Verification items for the finished model (mm, model axes). A direction names the side the tool comes from. Round coordinates to 2 decimals unless told otherwise and drop trailing zeros. Order: outer loops, then holes, each group sorted by start corner. A loop starts at its lowest first (then second) coordinate and runs counter-clockwise, first axis right, second up. Notation, with made-up numbers: (-11, 62.5) -> (-2, 62.5) arc R27 cw to (-2, 83.5) -> close; hole circle Ø5 at (40, 27.5). An arc over 180 degrees is marked (long way). Answer in a Markdown table with one row per item. Add a question column.
```python
from build123d import *

# Parameters (mm, degrees)
SKETCH2_R           = 6.35
BOSS_EXTRUDE1_DEPTH = 57.15
SKETCH4_W           = 69.85
SKETCH4_H           = 12.7
BOSS_EXTRUDE6_DEPTH = 12.7
SKETCH8_W           = 12.7
SKETCH8_H           = 12.7
BOSS_EXTRUDE7_DEPTH = 107.95
SKETCH9_R           = 6.35
BOSS_EXTRUDE8_DEPTH = 88.9


with BuildPart() as part:
    # Sketch2 → Boss-Extrude1 (new body)
    with BuildSketch(Plane(origin=(0, 0, 0), x_dir=(1, 0, 0), z_dir=(0, 1, 0))):
        with Locations(Location((0, 0, 0), (0, 0, 270))):
            Circle(SKETCH2_R)
    extrude(amount=-BOSS_EXTRUDE1_DEPTH)

    # Sketch4 → Boss-Extrude6 (add)
    with BuildSketch(Plane.XZ.offset(57.15)):
        with Locations((28.575, 0)):
            Rectangle(SKETCH4_W, SKETCH4_H)
    extrude(amount=BOSS_EXTRUDE6_DEPTH)

    # Sketch8 → Boss-Extrude7 (add)
    with BuildSketch(Plane.XZ.offset(69.85)):
        with Locations((57.15, 0)):
            Rectangle(SKETCH8_W, SKETCH8_H)
    extrude(amount=BOSS_EXTRUDE7_DEPTH)

    # Sketch9 → Boss-Extrude8 (add)
    with BuildSketch(Plane.ZY.offset(-50.8)):
        with Locations((0, -171.45)):
            Circle(SKETCH9_R)
    extrude(amount=BOSS_EXTRUDE8_DEPTH)


solid = part.part
```
1) Draft check along Y on faces 1 (the face through (57, -177.8, 0)), 2 (the face through (22, -69.85, 0)), 3 (the face through (6.97, -177.65, -1.38)), 4 (the face through (50.8, -176, -5)). Enter one of: +Y half, -Y half, draft (parallel to the pull), parting line (faces both ways), or undercut.
2) Depth check by flat-ended pin: P1, Ø1.9, axis at x = -3.5, z = -3.5, coming from the +Y side; P2, Ø4, axis at x = -26.5, z = -4, coming from the -Y side; P3, Ø3, axis at x = 2, z = -5, coming from the -Y side; P4, Ø1.5, axis at y = -49, z = -4, coming from the -X side. Enter the tip coordinate at first touch or a pass-through.
3) Tool access check on faces 5 (the face through (50.8, -176, 5)), 6 (the face through (-6.35, -63, 0)), 7 (the face through (-3.86, -28.17, -5.04)), 8 (the face through (-5, -57.15, -5)). Record the directions out of +Z, -Z, +X, -X, +Y, -Y that give a thin tool (end or side, any length) a straight path to the whole face; none if there is none.
4) Cross-section at C-C, the plane y = -44. Record the boundary of the cut face in (x, z), and give its area (3 significant figures).
5) Cross-section at B-B, the plane z = -4. Record the boundary of the cut face in (x, y).
6) Cross-section at D-D, the plane x = -11.5. Record the boundary of the cut face in (y, z).
7) Cross-section at A-A, the plane x = 31. Record the boundary of the cut face in (y, z).
8) Thickness scan on L1, parallel to X at y = -138, z = 1.75; L2, parallel to Y at x = 26, z = 5; L3, parallel to Y at x = 15.5, z = 1. Record the ranges inside material, lowest first. Write a range as [from, to].
Results below:
| question | item | result |
|---|---|---|
| 1 | face 1 | -Y half |
| 1 | face 2 | undercut |
| 1 | face 3 | undercut |
| 1 | face 4 | draft |
| 2 | P1 | y = 0 |
| 2 | P2 | y = -177.48 |
| 2 | P3 | y = -176.75 |
| 2 | P4 | x = -5.46 |
| 3 | face 5 | +Z, -X, -Y |
| 3 | face 6 | +Z, -Z, -X, +Y |
| 3 | face 7 | +Y |
| 3 | face 8 | -Z, -X, +Y |
| 4 | outline | circle Ø12.7 at (0, 0) |
| 4 | area | 127 mm² |
| 5 | outline | (-38.1, -176.38) -> (50.8, -176.38) -> (50.8, -177.8) -> (63.5, -177.8) -> (63.5, -57.15) -> (4.93, -57.15) -> (4.93, 0) -> (-4.93, 0) -> (-4.93, -57.15) -> (-6.35, -57.15) -> (-6.35, -69.85) -> (50.8, -69.85) -> (50.8, -166.52) -> (-38.1, -166.52) -> close |
| 6 | outline | circle Ø12.7 at (-171.45, 0) |
| 7 | outline | circle Ø12.7 at (-171.45, 0); (-69.85, -6.35) -> (-57.15, -6.35) -> (-57.15, 6.35) -> (-69.85, 6.35) -> close |
| 8 | L1 | [50.8, 63.5] |
| 8 | L2 | [-175.36, -167.54], [-69.85, -57.15] |
| 8 | L3 | [-177.72, -165.18], [-69.85, -57.15] |
